```python
from build123d import *

# Parameters (mm, degrees)
SKETCH1_W               = 44.45
SKETCH1_H               = 38.1
BOSS_EXTRUDE1_DEPTH     = 3.175
CUT_EXTRUDE1_DEPTH      = 49.464271634
CUT_EXTRUDE1_DEPTH_BACK = 49.464271634
SKETCH2_R               = 3.302
SKETCH3_W               = 3.175
SKETCH3_H               = 38.1
BOSS_EXTRUDE2_DEPTH     = 28.575
FILLET1_R               = 12.7


with BuildPart() as part:
    # Sketch1 → Boss-Extrude1 (new body)
    with BuildSketch(Plane.XY):
        with Locations((22.225, 0)):
            Rectangle(SKETCH1_W, SKETCH1_H)
    extrude(amount=BOSS_EXTRUDE1_DEPTH)

    # Sketch2 → Cut-Extrude1 (cut, two sides: drawn at the far end of the back side and taken through both)
    with BuildSketch(Plane.XY.offset(3.175).offset(-CUT_EXTRUDE1_DEPTH_BACK)):
        with Locations((30.48, 6.35)):
            Circle(SKETCH2_R)
        with Locations((30.48, -6.35)):
            Circle(SKETCH2_R)
    extrude(amount=CUT_EXTRUDE1_DEPTH + CUT_EXTRUDE1_DEPTH_BACK, mode=Mode.SUBTRACT)

    # Sketch3 → Boss-Extrude2 (add)
    with BuildSketch(Plane(origin=(0, 0, 0), x_dir=(-1, 0, 0), z_dir=(0, 0, -1))):
        with Locations((-1.5875, 0)):
            Rectangle(SKETCH3_W, SKETCH3_H)
    extrude(amount=BOSS_EXTRUDE2_DEPTH)

    # Fillet1
    fillet1_edges = [part.edges().sort_by_distance(p)[0] for p in [
        (44.45, 19.05, 1.5875),
        (44.45, -19.05, 1.5875),
    ]]
    fillet(fillet1_edges, radius=FILLET1_R)


solid = part.part
```
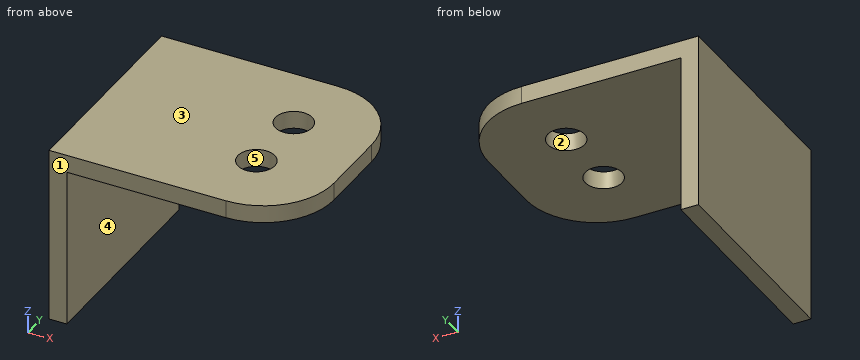
Geometry check sheet. Reference: the model listing, model coordinates, mm. Face numbers are marked on the shaded views. A direction names the side the tool comes from. Round coordinates to 2 decimals unless told otherwise and drop trailing zeros. Loops run counter-clockwise (first coordinate to the right, second up) from the corner with the lowest first, then second, coordinate; pieces in that order, holes last. Notation, with made-up numbers: M 66,0 L 80,0 A14 cw 80,20 Z; hole C -7.75,0.25 d7. An arc over 180 degrees is marked long. Return JSON: item names as keys, results as strings. Group by question number.
(1) Set-up check for the marked faces 4 and 5: record each of +Z, -Z, +X, -X, +Y, -Y from which the full face is reachable in a straight line by a thin tool's end or side.
(2) Mould release check, pull along Y, two halves, no side actions. Record for the marked faces 1, 2 and 3: pulls with the +Y half, pulls with the -Y half, needs draft (parallel to the pull), parting line crosses it, or undercut.
(3) Go/stop test with flat-tipped pins: pin 1 (7.5 mm diameter, centred on x = 30.48, y = 6.35, fed in from -Z); pin 2 (8 mm diameter, centred on y = 5.5, z = -12.5, fed in from +X) (3 decimals); pin 3 (6 mm diameter, centred on x = 29.5, y = -7, fed in from +Z) (3 decimals). Record where each tip stops, or that it passes through.
(4) Section check B-B, the plane y = -8.5. Enter the section's corners in (x, z) (3 decimals), and give its area (3 significant figures).
(5) Scan lines: line 1 along Y through (x, z) = (30.48, 1.4); line 2 along Y through (x, z) = (30, 2); line 3 along X through (y, z) = (-6.35, 1.4). Record each from-to range of solid material in increasing order. Write a range as [from, to].
(6) Section check A-A, the plane x = 30.48. Enter the section's corners in (y, z) (3 decimals).
(7) Section check D-D, the plane z = -13.5. Enter the section's corners in (x, y) (3 decimals), and give its area (3 significant figures).
(8) Section check C-C, the plane y = 1. Enter the section's corners in (x, z) (3 decimals).
Data:
{
 "1": {"face 4": "-Z, +X, +Y, -Y", "face 5": "+Z, -Z"},
 "2": {"face 1": "pulls with the -Y half", "face 2": "undercut", "face 3": "needs draft"},
 "3": {"pin 1": "z = 0", "pin 2": "x = 3.175", "pin 3": "z = 3.175"},
 "4": {"outline": "M 0,-28.575 L 3.175,-28.575 L 3.175,0 L 27.974,0 L 27.974,3.175 L 0,3.175 Z; M 32.986,0 L 44.267,0 L 44.267,3.175 L 32.986,3.175 Z", "area": "215 mm²"},
 "5": {"line 1": "[-19.05, -9.65], [-3.05, 3.05], [9.65, 19.05]", "line 2": "[-19.05, -9.62], [-3.08, 3.08], [9.62, 19.05]", "line 3": "[0, 27.18], [33.78, 44.45]"},
 "6": {"outline": "M -19.05,0 L -9.652,0 L -9.652,3.175 L -19.05,3.175 Z; M -3.048,0 L 3.048,0 L 3.048,3.175 L -3.048,3.175 Z; M 9.652,0 L 19.05,0 L 19.05,3.175 L 9.652,3.175 Z"},
 "7": {"outline": "M 0,-19.05 L 3.175,-19.05 L 3.175,19.05 L 0,19.05 Z", "area": "121 mm²"},
 "8": {"outline": "M 0,-28.575 L 3.175,-28.575 L 3.175,0 L 44.45,0 L 44.45,3.175 L 0,3.175 Z"}
}
